Autodesk Inventor part; units mm, degrees
ref_plane "YZ Plane" through (0, 0, 0) normal (1, 0, 0) x (0, 1, 0)
ref_plane "XZ Plane" through (0, 0, 0) normal (0, 1, 0) x (-1, 0, 0)
ref_plane "XY Plane" through (0, 0, 0) normal (0, 0, 1) x (1, 0, 0)
sketch "Эскиз1" plane through (0, 0, 0) normal (0, 0, 1) x (1, 0, 0)
  circle A0 centre (0, 0) radius 88.5486
  circle A1 centre (0, 0) radius 70 construction
  circle A2 centre (0, 70) radius 7.5
  circle A3 centre (0, 0) radius 70 construction
  circle A4 centre (-23.9414, 65.7785) radius 7.5
  circle A5 centre (0, 0) radius 70 construction
  circle A6 centre (-44.9951, 53.6231) radius 7.5
  circle A7 centre (0, 0) radius 70 construction
  circle A8 centre (-60.6218, 35) radius 7.5
  circle A9 centre (0, 0) radius 70 construction
  circle A10 centre (-68.9365, 12.1554) radius 7.5
  circle A11 centre (0, 0) radius 70 construction
  circle A12 centre (-68.9365, -12.1554) radius 7.5
  circle A13 centre (0, 0) radius 70 construction
  circle A14 centre (-60.6218, -35) radius 7.5
  circle A15 centre (0, 0) radius 70 construction
  circle A16 centre (-44.9951, -53.6231) radius 7.5
  circle A17 centre (0, 0) radius 70 construction
  circle A18 centre (-23.9414, -65.7785) radius 7.5
  circle A19 centre (0, 0) radius 70 construction
  circle A20 centre (0, -70) radius 7.5
  circle A21 centre (0, 0) radius 70 construction
  circle A22 centre (23.9414, -65.7785) radius 7.5
  circle A23 centre (0, 0) radius 70 construction
  circle A24 centre (44.9951, -53.6231) radius 7.5
  circle A25 centre (0, 0) radius 70 construction
  circle A26 centre (60.6218, -35) radius 7.5
  circle A27 centre (0, 0) radius 70 construction
  circle A28 centre (68.9365, -12.1554) radius 7.5
  circle A29 centre (0, 0) radius 70 construction
  circle A30 centre (68.9365, 12.1554) radius 7.5
  circle A31 centre (0, 0) radius 70 construction
  circle A32 centre (60.6218, 35) radius 7.5
  circle A33 centre (0, 0) radius 70 construction
  circle A34 centre (44.9951, 53.6231) radius 7.5
  circle A35 centre (0, 0) radius 70 construction
  circle A36 centre (23.9414, 65.7785) radius 7.5
  dimension "d0" = 140
  dimension "d1" = 15
  dimension "d4" = 360
extrude "Выдавливание1" add sketch "Эскиз1" against normal blind 15
chamfer "Фаска1" distance 2 angle 45 18 edges at (-31.4414, -65.7785, 0) (-7.5, -70, 0) (16.4414, -65.7785, 0) (37.4951, -53.6231, 0) (53.1218, -35, 0) (61.4365, -12.1554, 0) (61.4365, 12.1554, 0) (53.1218, 35, 0) (37.4951, 53.6231, 0) (16.4414, 65.7785, 0) (-7.5, 70, 0) (-31.4414, 65.7785, 0) (-52.4951, 53.6231, 0) (-68.1218, 35, 0) (-76.4365, 12.1554, 0) (-76.4365, -12.1554, 0) (-68.1218, -35, 0) (-52.4951, -53.6231, 0)
properties part number "Диск"
Here's how the part is built. I have some questions about the finished solid (model axes, mm). Give positions to 0.01 mm unless a question says otherwise; leave off trailing zeros. Order: outer loops, then holes, each group sorted by start corner. A loop starts at its lowest first (then second) coordinate and runs counter-clockwise, first axis right, second up. Notation, with made-up numbers: M 21.25,39 L 52.25,39 A34 ccw 52.25,78 Z; hole C 20,11.25 d4. An arc over 180 degrees is marked long. Answer as a JSON object with one key per item and string values. Group by question number.
1) I'm going to push flat-ended pins straight in: pin 1 Ø6 at (x, y) = (-42.5, -37) entering from +Z; pin 2 Ø4 at (y, z) = (16.5, -7.5) entering from +X; pin 3 Ø12 at (x, y) = (-23.94, -65.78) entering from -Z; pin 4 Ø1 at (x, z) = (23.5, -9) entering from -Y. Where does each tip first touch, or does it pass through?
2) Suppose I cut it at B-B, the plane z = -11.75. Count the separate pieces of the cut face and the enclosed holes in it, plus the area to 3 significant figures.
3) Please list where these lines run through material, in increasing order: L1, parallel to Y at x = 0, z = -6.25; L2, parallel to Y at x = -75.5, z = -6.25; L3, parallel to X at y = -58, z = -2.5. Write a range as [from, to].
4) Suppose I cut it at A-A, the plane x = 0. Write out the boundary of the cut face in (y, z).
5) Suppose I cut it at C-C, the plane y = -35. Write out the boundary of the cut face in (x, z), plus the area to 3 significant figures.
Results found:
{
 "1": {"pin 1": "z = 0", "pin 2": "x = 87.35", "pin 3": "through", "pin 4": "y = -85.51"},
 "2": {"separate pieces": "1", "enclosed holes": "18", "area": "21,500 mm²"},
 "3": {"L1": "[-88.55, -77.5], [-62.5, 62.5], [77.5, 88.55]", "L2": "[-46.27, -15.78], [-8.53, 8.53], [15.78, 46.27]", "L3": "[-66.91, -51.09], [-38.9, 38.9], [51.09, 66.91]"},
 "4": {"outline": "M -88.55,-15 L -77.5,-15 L -77.5,-2 L -79.5,0 L -88.55,0 Z; M -62.5,-15 L 62.5,-15 L 62.5,-2 L 60.5,0 L -60.5,0 L -62.5,-2 Z; M 77.5,-15 L 88.55,-15 L 88.55,0 L 79.5,0 L 77.5,-2 Z"},
 "5": {"outline": "M -81.34,-15 L -68.12,-15 L -68.12,-2 L -70.12,0 L -81.34,0 Z; M -53.12,-15 L 53.12,-15 L 53.12,-2 L 51.12,0 L -51.12,0 L -53.12,-2 Z; M 68.12,-15 L 81.34,-15 L 81.34,0 L 70.12,0 L 68.12,-2 Z", "area": "1,980 mm²"}
}
